from build123d import *

# Parameters (mm, degrees)
SKETCH_1_R      = 15.5
EXTRUDE_1_DEPTH = 16


with BuildPart() as part:
    # 草图1 → 拉伸1 (new body)
    with BuildSketch(Plane.XY):
        Polygon((380.780090503, 350), (-39.219909497, 350), (-39.219909497, 0), (20.780090503, -300), (320.780090503, -300), (380.780090503, 0), align=None)
        with Locations((75.780090503, -255)):
            Circle(SKETCH_1_R, mode=Mode.SUBTRACT)
        with Locations((75.780090503, -55)):
            Circle(SKETCH_1_R, mode=Mode.SUBTRACT)
        with Locations((75.780090503, -155)):
            Circle(SKETCH_1_R, mode=Mode.SUBTRACT)
        with Locations((110.780090503, 80)):
            Circle(SKETCH_1_R, mode=Mode.SUBTRACT)
        with Locations((10.780090503, 80)):
            Circle(SKETCH_1_R, mode=Mode.SUBTRACT)
        with Locations(Location((110.780090503, 270, 0), (0, 0, 180))):
            Circle(SKETCH_1_R, mode=Mode.SUBTRACT)
        with Locations(Location((10.780090503, 270, 0), (0, 0, 180))):
            Circle(SKETCH_1_R, mode=Mode.SUBTRACT)
        with Locations((330.780090503, 270)):
            Circle(SKETCH_1_R, mode=Mode.SUBTRACT)
        with Locations((230.780090503, 270)):
            Circle(SKETCH_1_R, mode=Mode.SUBTRACT)
        with Locations(Location((330.780090503, 80, 0), (0, 0, 180))):
            Circle(SKETCH_1_R, mode=Mode.SUBTRACT)
        with Locations(Location((230.780090503, 80, 0), (0, 0, 180))):
            Circle(SKETCH_1_R, mode=Mode.SUBTRACT)
        with Locations(Location((265.780090503, -155, 0), (0, 0, 180))):
            Circle(SKETCH_1_R, mode=Mode.SUBTRACT)
        with Locations(Location((265.780090503, -55, 0), (0, 0, 180))):
            Circle(SKETCH_1_R, mode=Mode.SUBTRACT)
        with Locations(Location((265.780090503, -255, 0), (0, 0, 180))):
            Circle(SKETCH_1_R, mode=Mode.SUBTRACT)
    extrude(amount=EXTRUDE_1_DEPTH)


solid = part.part
Geometry check sheet. Reference: the model listing, model coordinates, mm. Give positions to 0.01 mm unless a question says otherwise; leave off trailing zeros. Order: outer loops, then holes, each group sorted by start corner. A loop starts at its lowest first (then second) coordinate and runs counter-clockwise, first axis right, second up.
1) Cross-section at B-B (y = 80). Record the boundary of the cut face in (x, z).
Results are:
outline: (-39.22, 0) - (-4.72, 0) - (-4.72, 16) - (-39.22, 16) - close; (26.28, 0) - (95.28, 0) - (95.28, 16) - (26.28, 16) - close; (126.28, 0) - (215.28, 0) - (215.28, 16) - (126.28, 16) - close; (246.28, 0) - (315.28, 0) - (315.28, 16) - (246.28, 16) - close; (346.28, 0) - (380.78, 0) - (380.78, 16) - (346.28, 16) - close
2) Cross-section at D-D (y = -255). Record the boundary of the cut face in (x, z), then the cut area to 3 significant figures.
Results are:
outline: (11.78, 0) - (60.28, 0) - (60.28, 16) - (11.78, 16) - close; (91.28, 0) - (250.28, 0) - (250.28, 16) - (91.28, 16) - close; (281.28, 0) - (329.78, 0) - (329.78, 16) - (281.28, 16) - close
area: 4,100 mm2
3) Draft check along X on faces 1 (the flat face through (350.36, -152.1, 7.89)), 2 (the cylindrical face through (245.564, 274.656, 7.888)), 3 (the flat face through (174, 350, 8)), 4 (the cylindrical face through (257.45, -268.07, 7.89)). Enter one of: released by +X, released by -X, zero draft, split by the parting line, or undercut.
Results are:
face 1: released by +X
face 2: undercut
face 3: zero draft
face 4: undercut
4) Cross-section at C-C (x = 103). Record the boundary of the cut face in (y, z), then the cut area to 3 significant figures.
Results are:
outline: (-300, 0) - (66.59, 0) - (66.59, 16) - (-300, 16) - close; (93.41, 0) - (256.59, 0) - (256.59, 16) - (93.41, 16) - close; (283.41, 0) - (350, 0) - (350, 16) - (283.41, 16) - close
area: 9,540 mm2
5) Material ranges on probe 1 along X at (y, z) = (279, 15); probe 2 along Y at (x, z) = (122.5, 5); probe 3 along Y at (x, z) = (121, 3.75), recorded low to high.
Results are:
probe 1: x = -39.22 to -1.84, 23.4 to 98.16, 123.4 to 218.16, 243.4 to 318.16, 343.4 to 380.78
probe 2: y = -300 to 69.86, 90.14 to 259.86, 280.14 to 350
probe 3: y = -300 to 68.35, 91.65 to 258.35, 281.65 to 350
6) Cross-section at A-A (z = 4). Give the number of separate pieces and of enclosed holes in the cut face, then the cut area to 3 significant figures.
Results are:
separate pieces: 1
enclosed holes: 14
area: 244,000 mm2
7) Gauge pin test, flat end, axial feed: pin 1 (4 mm diameter, centred on y = -106, z = 2.5, fed in from -X). Record the tip position at first contact, or that the pin passes through.
Results are:
pin 1: stops at x = -18.42
